from build123d import *

# Parameters (mm, degrees)
F0_W     = 40
F0_H     = 40
F1_DEPTH = 3


with BuildPart() as f1:
    # F0 (on Top) → F1 (new body)
    with BuildSketch(Plane.XY):
        Rectangle(F0_W, F0_H)
        Polygon((-12.221825, -7.272078), (-7.272078, -12.221825), (-12.221825, -17.171573), (-17.171573, -12.221825), align=None, mode=Mode.SUBTRACT)
        Polygon((7.272078, -12.221825), (12.221825, -7.272078), (17.171573, -12.221825), (12.221825, -17.171573), align=None, mode=Mode.SUBTRACT)
        Polygon((-12.221825, 7.272078), (-17.171573, 12.221825), (-12.221825, 17.171573), (-7.272078, 12.221825), align=None, mode=Mode.SUBTRACT)
        Polygon((12.221825, 7.272078), (7.272078, 12.221825), (12.221825, 17.171573), (17.171573, 12.221825), align=None, mode=Mode.SUBTRACT)
    extrude(amount=F1_DEPTH)


solid = f1.part
Input: part model. Units: mm. Frame: model coordinates. A direction names the side the tool comes from. Give positions to 0.01 mm unless a question says otherwise; leave off trailing zeros. Order: outer loops, then holes, each group sorted by start corner. A loop starts at its lowest first (then second) coordinate and runs counter-clockwise, first axis right, second up. Notation, with made-up numbers: (42, 9.25) - (73, 9.25) arc R34 ccw to (73, 47.25) - close; hole circle Ø8 at (-18, 35). An arc over 180 degrees is marked (long way). Answer as a JSON object with one key per item and string values. Group by question number.
Q1. Line query: probe 1 along X at (y, z) = (-15, 2.75); probe 2 along X at (y, z) = (9, 2.85); probe 3 along Y at (x, z) = (-16.5, 1.7). Output: solid intervals per line, ascending.
Q2. Set-up query: faces 1 (the face through (0, 0, 3)), 2 (the face through (-9.712, 9.782, 1.479)). Return all of +Z, -Z, +X, -X, +Y, -Y with unobstructed straight access to the full face (end or side cutting, diameter ignored); none if empty.
Q3. Mould query, pull axis Y, two halves, no side actions, for faces 3 (the face through (14.662, 14.731, 1.479)), 4 (the face through (9.71, 14.66, 1.48)), 5 (the face through (-20, 0, 1)), 6 (the face through (0, -20, 1)). Classes: pulls with the +Y half, pulls with the -Y half, needs draft (parallel to the pull), parting line crosses it, or undercut.
Q4. Cut plane B-B, the plane y = 8. Output: boundary loops of the cut face in (x, z).
Q5. Cut plane A-A, the plane z = 2.55. Output: boundary loops of the cut face in (x, y), then the cut area to 3 significant figures.
Q6. Cut plane C-C, the plane x = 11. Output: boundary loops of the cut face in (y, z).
Results:
{
 "1": {"probe 1": "-20 to -14.39, -10.05 to 10.05, 14.39 to 20", "probe 2": "-20 to -13.95, -10.49 to 10.49, 13.95 to 20", "probe 3": "-20 to -12.89, -11.55 to 11.55, 12.89 to 20"},
 "2": {"face 1": "+Z, +X, -X, +Y, -Y", "face 2": "+Z, -Z"},
 "3": {"face 3": "undercut", "face 4": "undercut", "face 5": "needs draft", "face 6": "pulls with the -Y half"},
 "4": {"outline": "(-20, 0) - (-12.95, 0) - (-12.95, 3) - (-20, 3) - close; (-11.49, 0) - (11.49, 0) - (11.49, 3) - (-11.49, 3) - close; (12.95, 0) - (20, 0) - (20, 3) - (12.95, 3) - close"},
 "5": {"outline": "(-20, -20) - (20, -20) - (20, 20) - (-20, 20) - close; hole (-17.17, -12.22) - (-12.22, -17.17) - (-7.27, -12.22) - (-12.22, -7.27) - close; hole (-17.17, 12.22) - (-12.22, 7.27) - (-7.27, 12.22) - (-12.22, 17.17) - close; hole (7.27, -12.22) - (12.22, -17.17) - (17.17, -12.22) - (12.22, -7.27) - close; hole (7.27, 12.22) - (12.22, 7.27) - (17.17, 12.22) - (12.22, 17.17) - close", "area": "1,400 mm^2"},
 "6": {"outline": "(-20, 0) - (-15.95, 0) - (-15.95, 3) - (-20, 3) - close; (-8.49, 0) - (8.49, 0) - (8.49, 3) - (-8.49, 3) - close; (15.95, 0) - (20, 0) - (20, 3) - (15.95, 3) - close"}
}
